Check sheet for the modelled part. Datum: model origin and axes. Units: mm. Round coordinates to 2 decimals unless told otherwise and drop trailing zeros. Answer in a Markdown table with one row per item. Add a question column.
1. Material ranges on L1, parallel to X at y = 471, z = 27.5; L2, parallel to X at y = 475, z = 19; L3, parallel to Z at x = 13.5, y = 468.5, recorded low to high. Write a range as from..to.
2. Sectioned sample at A-A, the plane y = 474. Count the separate pieces of the cut face and the enclosed holes in it, then the cut area to 3 significant figures.
3. Draft check along Y on faces 1 (the cylindrical face through (22.944, 464.142, 27.095)), 2 (the cylindrical face through (44.083, 476.67, 20.188)). Enter one of: +Y half, -Y half, draft (parallel to the pull), parting line (faces both ways), or undercut.
4. Depth check by flat-ended pin: P1, Ø6, axis at y = 480, z = 50, coming from the -X side; P2, Ø6, axis at y = 461.5, z = 43.5, coming from the -X side; P3, Ø12, axis at y = 478.5, z = 36.5, coming from the -X side. Enter the tip coordinate at first touch or a pass-through.
```python
from build123d import *

# Parameters (mm, degrees)
BOSS_EXTRUDE2_DEPTH      = 12
BOSS_EXTRUDE2_DEPTH_BACK = 18.35
SKETCH3_R                = 20.599499999
CUT_EXTRUDE2_DEPTH       = 10
SKETCH5_R                = 30.999999999
BOSS_EXTRUDE3_DEPTH      = 10
CUT_EXTRUDE3_REACH       = 100.809
SKETCH7_R                = 1.365


with BuildPart() as part:
    # Sketch3 → Boss-Extrude2 (new, two sides: drawn at the far end of the back side and taken through both)
    with BuildSketch(Plane(origin=(53.132442303, 452.346775715, 5.622561963), x_dir=(0.9931732430561937, -0.11663964741431751, -0.0014498028509745849), z_dir=(-0.11664865741723304, -0.9930965298387961, -0.012343951753720052)).offset(-BOSS_EXTRUDE2_DEPTH_BACK)):
        with Locations(Location((-41.42738807, 23.530711727, 0), (0, 0, 180.083073943))):
            Circle(SKETCH3_R)
    extrude(amount=BOSS_EXTRUDE2_DEPTH + BOSS_EXTRUDE2_DEPTH_BACK)

    # Sketch4 → Cut-Extrude2 (cut)
    with BuildSketch(Plane(origin=(51.732658414, 440.429617357, 5.474434542), x_dir=(0.9931732430561937, -0.1166396474143174, -0.001449802850974575), z_dir=(-0.11664865741723293, -0.9930965298387961, -0.012343951753719985))):
        with BuildLine():
            Line((-38.551989149, 22.67509438), (-41.097444518, 20.548910719))
            ThreePointArc((-41.097444518, 20.548910719), (-44.186998686, 22.354043021), (-43.350593551, 25.833162742))
            ThreePointArc((-43.350593551, 25.833162742), (-39.778140656, 26.036701146), (-38.551989149, 22.67509438))
        make_face()
    extrude(amount=-CUT_EXTRUDE2_DEPTH, mode=Mode.SUBTRACT)

    # Sketch5 → Boss-Extrude3 (add)
    with BuildSketch(Plane(origin=(55.272945167, 470.570097038, 5.849073478), x_dir=(0.9931732430561937, -0.11663964741431687, -0.0014498028509745493), z_dir=(0.11664865741723239, 0.9930965298387961, 0.012343951753719856))):
        with Locations(Location((-41.42738807, -23.530711727, 0), (0, 0, 359.916926057))):
            Circle(SKETCH5_R)
    extrude(amount=BOSS_EXTRUDE3_DEPTH)

    # Sketch7 → Cut-Extrude3 (cut, up to next)
    with BuildSketch(Plane(origin=(56.439431742, 480.501062336, 5.972512996), x_dir=(0.9931732430561937, -0.11663964741431691, -0.0014498028509745543), z_dir=(0.11664865741723243, 0.9930965298387961, 0.012343951753719861)), mode=Mode.PRIVATE) as cut_extrude3_sk1:
        with Locations(Location((-40.55325276, -33.270564316, 0), (0, 0, 179.916926057))):
            Circle(SKETCH7_R)
    cut_extrude3_tool1 = extrude(cut_extrude3_sk1.sketch, amount=-CUT_EXTRUDE3_REACH, mode=Mode.PRIVATE) & part.part
    # Sketch7 → Cut-Extrude3 (cut, up to next)
    with BuildSketch(Plane(origin=(56.439431742, 480.501062336, 5.972512996), x_dir=(0.9931732430561937, -0.11663964741431691, -0.0014498028509745543), z_dir=(0.11664865741723243, 0.9930965298387961, 0.012343951753719861)), mode=Mode.PRIVATE) as cut_extrude3_sk2:
        with Locations(Location((-51.16724066, -24.404847037, 0), (0, 0, 179.916926057))):
            Circle(SKETCH7_R)
    cut_extrude3_tool2 = extrude(cut_extrude3_sk2.sketch, amount=-CUT_EXTRUDE3_REACH, mode=Mode.PRIVATE) & part.part
    # Sketch7 → Cut-Extrude3 (cut, up to next)
    with BuildSketch(Plane(origin=(56.439431742, 480.501062336, 5.972512996), x_dir=(0.9931732430561937, -0.11663964741431691, -0.0014498028509745543), z_dir=(0.11664865741723243, 0.9930965298387961, 0.012343951753719861)), mode=Mode.PRIVATE) as cut_extrude3_sk3:
        with Locations(Location((-42.301523381, -13.790859137, 0), (0, 0, 179.916926057))):
            Circle(SKETCH7_R)
    cut_extrude3_tool3 = extrude(cut_extrude3_sk3.sketch, amount=-CUT_EXTRUDE3_REACH, mode=Mode.PRIVATE) & part.part
    # Sketch7 → Cut-Extrude3 (cut, up to next)
    with BuildSketch(Plane(origin=(56.439431742, 480.501062336, 5.972512996), x_dir=(0.9931732430561937, -0.11663964741431691, -0.0014498028509745543), z_dir=(0.11664865741723243, 0.9930965298387961, 0.012343951753719861)), mode=Mode.PRIVATE) as cut_extrude3_sk4:
        with Locations(Location((-31.687535481, -22.656576416, 0), (0, 0, 179.916926057))):
            Circle(SKETCH7_R)
    cut_extrude3_tool4 = extrude(cut_extrude3_sk4.sketch, amount=-CUT_EXTRUDE3_REACH, mode=Mode.PRIVATE) & part.part
    add(cut_extrude3_tool1.solids().sort_by_distance((16.163026, 484.817666, 39.299302))[0], mode=Mode.SUBTRACT)
    add(cut_extrude3_tool2.solids().sort_by_distance((5.621497, 486.165868, 30.449657))[0], mode=Mode.SUBTRACT)
    add(cut_extrude3_tool3.solids().sort_by_distance((14.426691, 485.263693, 19.823636))[0], mode=Mode.SUBTRACT)
    add(cut_extrude3_tool4.solids().sort_by_distance((24.968219, 483.915491, 28.67328))[0], mode=Mode.SUBTRACT)


solid = part.part
```
Answer key:
| question | item | result |
|---|---|---|
| 1 | L1 | x = -7.01..22.53, 24.37..34.3 |
| 1 | L2 | x = -3.78..12.04, 14.4..43.49 |
| 1 | L3 | z = 8.76..18.73, 20.51..37.95, 40.24..49.96 |
| 2 | separate pieces | 1 |
| 2 | enclosed holes | 4 |
| 2 | area | 1,960 mm² |
| 3 | face 1 | undercut |
| 3 | face 2 | parting line |
| 4 | P1 | stops at x = -11.06 |
| 4 | P2 | stops at x = -4.87 |
| 4 | P3 | stops at x = -16.64 |
